Input: part model. Units: mm. Frame: model coordinates. A direction names the side the tool comes from. Coordinates: 2 decimals unless noted, no trailing zeros. Loops run counter-clockwise (first coordinate to the right, second up) from the corner with the lowest first, then second, coordinate; pieces in that order, holes last.
```python
from build123d import *

# Parameters (mm, degrees)
BOSS_EXTRUDE1_DEPTH                               = 38.1
SKETCH1_W                                         = 6.35
SKETCH1_H                                         = 16.002
BOSS_EXTRUDE1_2_DEPTH                             = 38.1
SKETCH1_4_W                                       = 144.018
SKETCH1_4_H                                       = 41.402
BOSS_EXTRUDE2_DEPTH                               = 6.35
SKETCH1_5_W                                       = 131.318
SKETCH1_5_H                                       = 6.35
BOSS_EXTRUDE3_DEPTH                               = 38.1
CSK_FOR_8_FLAT_HEAD_MACHINE_SCREW_100_D           = 4.4958
CSK_FOR_8_FLAT_HEAD_MACHINE_SCREW_100_CSINK_D     = 8.4328
CSK_FOR_8_FLAT_HEAD_MACHINE_SCREW_100_CSINK_ANGLE = 100
BOSS_EXTRUDE6_DEPTH                               = 6.35
CUT_EXTRUDE3_DEPTH                                = 105.525006773
CUT_EXTRUDE3_DEPTH_BACK                           = 105.525006773
BOSS_EXTRUDE7_DEPTH                               = 6.35


with BuildPart() as part:
    # Sketch1 → Boss-Extrude1 (new body)
    with BuildSketch(Plane(origin=(0, 0, 0), x_dir=(1, 0, 0), z_dir=(0, 1, 0))):
        Polygon((74.562549316, 16.479821782), (74.562549316, 10.129821782), (74.562549316, -31.272178218), (74.562549316, -37.622178218), (80.912549316, -37.622178218), (80.912549316, 16.479821782), align=None)
    extrude(amount=BOSS_EXTRUDE1_DEPTH)



with BuildPart() as body_2:
    # Sketch1 → Boss-Extrude1 2 (new body)
    with BuildSketch(Plane(origin=(0, 0, 0), x_dir=(1, 0, 0), z_dir=(0, 1, 0))):
        with Locations((-72.630450684, -10.571178218)):
            Rectangle(SKETCH1_W, SKETCH1_H)
    extrude(amount=BOSS_EXTRUDE1_2_DEPTH)


with BuildPart() as part_1:
    add(part.part)

    add(body_2.part)  # Boss-Extrude2 merges body 2
    # Sketch1_4 → Boss-Extrude2 (add)
    with BuildSketch(Plane(origin=(0, 0, 0), x_dir=(1, 0, 0), z_dir=(0, 1, 0))):
        with Locations((2.553549316, -10.571178218)):
            Rectangle(SKETCH1_4_W, SKETCH1_4_H)
    extrude(amount=BOSS_EXTRUDE2_DEPTH)

    # Sketch1_5 → Boss-Extrude3 (add)
    with BuildSketch(Plane(origin=(0, 0, 0), x_dir=(1, 0, 0), z_dir=(0, 1, 0))):
        with Locations((8.903549316, 13.304821782)):
            Rectangle(SKETCH1_5_W, SKETCH1_5_H)
        with Locations((8.903549316, -34.447178218)):
            Rectangle(SKETCH1_5_W, SKETCH1_5_H)
    extrude(amount=BOSS_EXTRUDE3_DEPTH)

    # CSK for _8 Flat Head Machine Screw _100 (through all)
    with Locations(Plane(origin=(0, 6.35, 0), x_dir=(1, 0, 0), z_dir=(0, 1, 0))):
        with Locations((-45.134950684, -21.937678218), (-45.134950684, 0.922321782), (50.115049316, 0.858821782), (50.115049316, -22.001178218)):
            CounterSinkHole(CSK_FOR_8_FLAT_HEAD_MACHINE_SCREW_100_D / 2, CSK_FOR_8_FLAT_HEAD_MACHINE_SCREW_100_CSINK_D / 2, counter_sink_angle=CSK_FOR_8_FLAT_HEAD_MACHINE_SCREW_100_CSINK_ANGLE)

    # Sketch1_8 → Boss-Extrude6 (add)
    with BuildSketch(Plane(origin=(0, 0, 0), x_dir=(1, 0, 0), z_dir=(0, 1, 0))):
        Polygon((-69.455450684, -31.272178218), (-69.455450684, -18.572178218), (-75.805450684, -18.572178218), (-75.805450684, -31.272178218), (-75.805450684, -37.622178218), (-56.755450684, -37.622178218), (-56.755450684, -31.272178218), align=None)
    extrude(amount=BOSS_EXTRUDE6_DEPTH)

    # Sketch11 → Cut-Extrude3 (cut, two sides: drawn at the far end of the back side and taken through both)
    with BuildSketch(Plane.XY.offset(37.622178218).offset(-CUT_EXTRUDE3_DEPTH_BACK)):
        with BuildLine():
            Line((-28.029969106, 38.1), (36.462549316, 38.1))
            ThreePointArc((36.462549316, 38.1), (4.216290105, 24.743162099), (-28.029969106, 38.1))
        make_face()
    extrude(amount=CUT_EXTRUDE3_DEPTH + CUT_EXTRUDE3_DEPTH_BACK, mode=Mode.SUBTRACT)

    # Sketch1_9 → Boss-Extrude7 (add)
    with BuildSketch(Plane(origin=(0, 0, 0), x_dir=(1, 0, 0), z_dir=(0, 1, 0))):
        Polygon((-69.455450684, -2.570178218), (-69.455450684, 10.129821782), (-56.755450684, 10.129821782), (-56.755450684, 16.479821782), (-69.455450684, 16.479821782), (-75.805450684, 16.479821782), (-75.805450684, 10.129821782), (-75.805450684, -2.570178218), align=None)
    extrude(amount=BOSS_EXTRUDE7_DEPTH)


solid = part_1.part
```
Item 1: Section query B-B (z = 16). Output: boundary loops of the cut face in (x, y).
Result:
outline: (-75.81, 0) - (80.91, 0) - (80.91, 38.1) - (74.56, 38.1) - (74.56, 6.35) - (-69.46, 6.35) - (-69.46, 38.1) - (-75.81, 38.1) - close
Item 2: Section query C-C (y = 30.5). Output: boundary loops of the cut face in (x, z), then the cut area to 3 significant figures.
Result:
outline: (-75.81, 2.57) - (-69.46, 2.57) - (-69.46, 18.57) - (-75.81, 18.57) - close; (-56.76, -16.48) - (-17.96, -16.48) - (-17.96, -10.13) - (-56.76, -10.13) - close; (-56.76, 31.27) - (-17.96, 31.27) - (-17.96, 37.62) - (-56.76, 37.62) - close; (26.4, -16.48) - (80.91, -16.48) - (80.91, 37.62) - (26.4, 37.62) - (26.4, 31.27) - (74.56, 31.27) - (74.56, -10.13) - (26.4, -10.13) - close
area: 1,550 mm2
Item 3: Mould query, pull axis Z, two halves, no side actions, for faces 6 (the face through (74.563, 22, 10)), 7 (the face through (-73, 22, 2.57)), 8 (the face through (1, 0, 10)). Classes: +Z half, -Z half, draft (parallel to the pull), parting line (faces both ways), or undercut.
Result:
face 6: undercut
face 7: -Z half
face 8: draft
Item 4: Line query: L1, parallel to Z at x = 44.5, y = 16; L2, parallel to X at y = 12, z = 8.5; L3, parallel to X at y = 24, z = 25.5. Output: solid intervals per line, ascending.
Result:
L1: z = -16.48 to -10.13, 31.27 to 37.62
L2: x = -75.81 to -69.46, 74.56 to 80.91
L3: x = 74.56 to 80.91
Item 5: Section query A-A (y = 8). Output: boundary loops of the cut face in (x, z).
Result:
outline: (-75.81, 2.57) - (-69.46, 2.57) - (-69.46, 18.57) - (-75.81, 18.57) - close; (-56.76, -16.48) - (80.91, -16.48) - (80.91, 37.62) - (-56.76, 37.62) - (-56.76, 31.27) - (74.56, 31.27) - (74.56, -10.13) - (-56.76, -10.13) - close
Item 6: Contact query for flat-ended pins moving along their axis: P1, Ø2, axis at y = 30, z = 20.5, coming from the -X side; P2, Ø1.9, axis at x = -73, y = 28, coming from the -Z side; P3, Ø6, axis at x = 50.12, z = 22, coming from the -Y side; P4, Ø10, axis at x = -3.5, y = 33, coming from the +Z side. Output: stop coordinate, or through.
Result:
P1: stops at x = 74.56
P2: stops at z = 2.57
P3: stops at y = 0
P4: passes through
Item 7: Section query D-D (x = 33.5). Output: boundary loops of the cut face in (y, z), then the cut area to 3 significant figures.
Result:
outline: (0, -16.48) - (35.39, -16.48) - (35.39, -10.13) - (6.35, -10.13) - (6.35, 31.27) - (35.39, 31.27) - (35.39, 37.62) - (0, 37.62) - close
area: 712 mm2
Item 8: Reachability of faces 1 (the face through (-56.755, 22, -13)), 2 (the face through (-73, 22, 18.572)), 3 (the face through (75, 38.1, 10)), 4 (the face through (8, 18, 31.272)), 5 (the face through (-69.455, 22, 11)) from +Z, -Z, +X, -X, +Y, -Y: full face, straight path, thin tool, end or side. Return the list, or none.
Result:
face 1: +Z, -Z, -X, +Y
face 2: +Z, -X, +Y
face 3: +Z, -Z, +X, -X, +Y
face 4: -X, +Y
face 5: +Z, -Z, +Y
